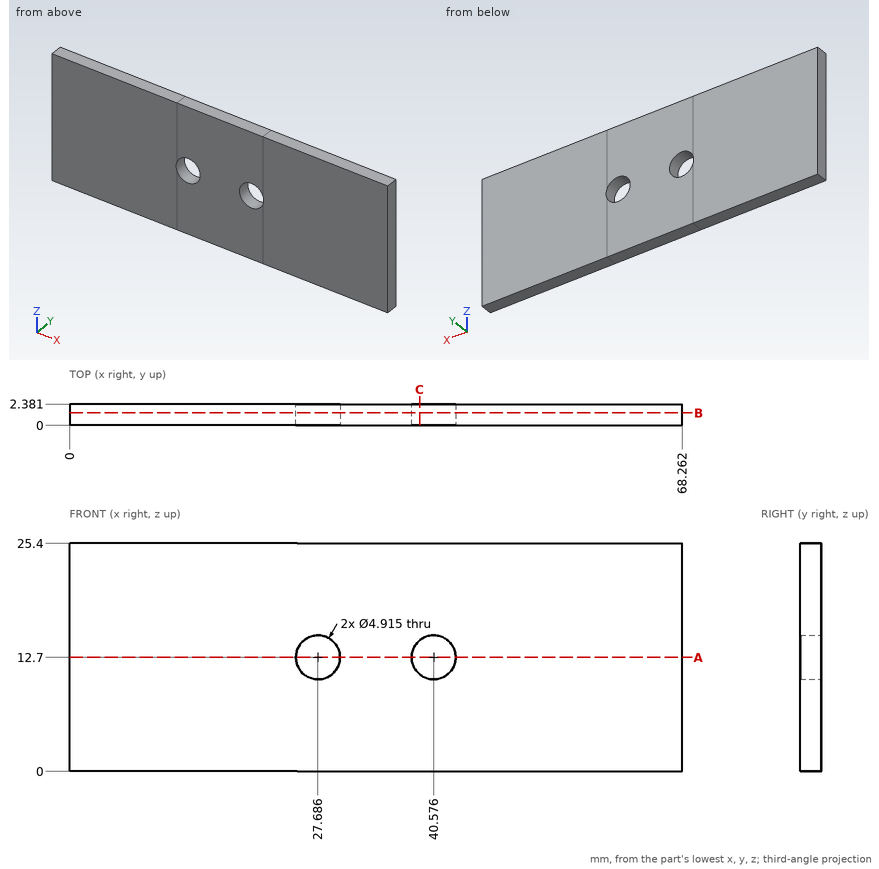
Print and shaded views of the part. All mm, measured from the part's lowest x, y and z. Give positions to 0.01 mm unless a question says otherwise; leave off trailing zeros. Loops run counter-clockwise (first coordinate to the right, second up) from the corner with the lowest first, then second, coordinate; pieces in that order, holes last. Notation, with made-up numbers: (64, 36) - (109, 36) arc R30 ccw to (109, 64) - close; hole circle Ø4 at (-18.5, 5.25). An arc over 180 degrees is marked (long way). One line per item, written item: value. Start each with the question number.
1. Slice it at A-A (z = 12.7). List the corners of the cut face in (x, y).
2. Pin check, flat tips, straight feed: pin 1 (1 mm diameter, centred on y = 1.5, z = 12.5, fed in from -X); pin 2 (4.5 mm diameter, centred on x = 40.58, z = 12.7, fed in from -Y). Stop position of each tip, or through.
3. Probe L1, parallel to X at y = 1.6, z = 12.7; L2, parallel to X at y = 1.75, z = 14; L3, parallel to Z at x = 39, y = 0.3 (1 decimal). List the from-to ranges inside material, lowest first. Write a range as from..to.
4. Slice it at B-B (y = 1.4). List the corners of the cut face in (x, z) (1 decimal), plus the area to 3 significant figures.
5. Slice it at C-C (x = 39). List the corners of the cut face in (y, z) (1 decimal).
Solution:
1. outline: (0, 0) - (25.23, 0) - (25.23, 2.38) - (0, 2.38) - close; (30.14, 0) - (38.12, 0) - (38.12, 2.38) - (30.14, 2.38) - close; (43.03, 0) - (68.26, 0) - (68.26, 2.38) - (43.03, 2.38) - close
2. pin 1: stops at x = 0
2. pin 2: passes through
3. L1: x = 0..25.23, 30.14..38.12, 43.03..68.26
3. L2: x = 0..25.6, 29.77..38.49, 42.66..68.26
3. L3: z = 0..10.8, 14.6..25.4
4. outline: (0, 0) - (68.3, 0) - (68.3, 25.4) - (0, 25.4) - close; hole circle Ø4.9 at (27.7, 12.7); hole circle Ø4.9 at (40.6, 12.7)
4. area: 1,700 mm^2
5. outline: (0, 0) - (2.4, 0) - (2.4, 10.8) - (0, 10.8) - close; (0, 14.6) - (2.4, 14.6) - (2.4, 25.4) - (0, 25.4) - close
